The listing builds one solid part. Answer for the finished solid, in the listing's coordinates (mm). Face numbers are marked on the shaded views. A direction names the side the tool comes from. Coordinates: 2 decimals unless noted, no trailing zeros. Write each loop counter-clockwise with the first axis right and the second up, starting at its lowest first coordinate (ties: lowest second). Pieces come first, ordered by that corner, then holes.
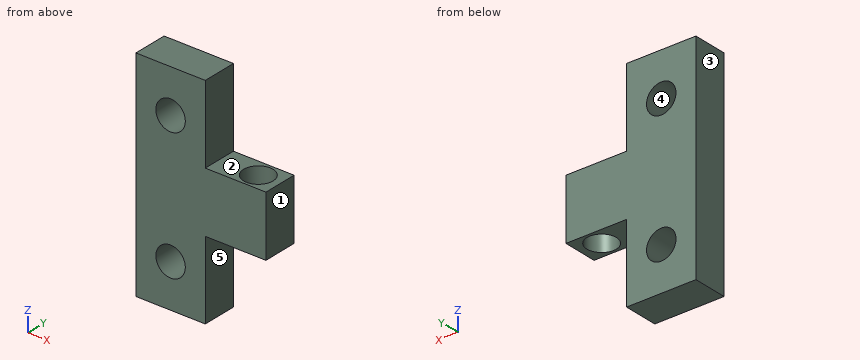
Autodesk Inventor part; units mm, degrees
ref_plane "YZ Plane" through (0, 0, 0) normal (1, 0, 0) x (0, 1, 0)
ref_plane "XZ Plane" through (0, 0, 0) normal (0, 1, 0) x (-1, 0, 0)
ref_plane "XY Plane" through (0, 0, 0) normal (0, 0, 1) x (1, 0, 0)
sketch "Skizze1" plane through (0, 0, 0) normal (0, 1, 0) x (-1, 0, 0)
  line L0 (0, 0) -> (15, 0)
  line L1 (15, 0) -> (15, -25)
  line L2 (15, -25) -> (0, -25)
  line L3 (0, -25) -> (0, 0)
  dimension "d0" = 25
  dimension "d1" = 15
extrude "Extrusion1" add sketch "Skizze1" along normal blind 4
sketch "Skizze3" plane through (0, 0, -25) normal (0, 0, -1) x (-1, 0, 0)
  point P0 (0, 0)
sketch "Skizze6" plane through (0, 4, 0) normal (0, 1, 0) x (1, 0, 0)
  circle A0 centre (-11, 5) radius 1.7
  line L0 (-15, 25) -> (-15, 0)
  line L1 (-15, 0) -> (0, 0)
  circle A1 centre (-11, 20) radius 1.7
  line L2 (0, 25) -> (-15, 25)
  point P0 (0, 30)
  dimension "d11" = 3.4
  dimension "d12" = 4
  dimension "d13" = 5
  dimension "d14" = 3.4
  dimension "d15" = 4
  dimension "d16" = 5
extrude "Extrusion4" cut sketch "Skizze6" against normal blind 30
sketch "Skizze7" plane through (0, 0, 0) normal (0, -1, 0) x (1, 0, 0)
  line L0 (0, -25) -> (-15, -25)
  line L1 (0, -25) -> (-7, -25)
  line L2 (-7, -25) -> (-7, -16)
  line L3 (-7, -16) -> (0, -16)
  line L4 (0, -16) -> (0, -25)
  line L5 (-15, 0) -> (0, 0)
  line L6 (0, 0) -> (-7, 0)
  line L7 (-7, 0) -> (-7, -9)
  line L8 (-7, -9) -> (0, -9)
  line L9 (0, -9) -> (0, 0)
  dimension "d19" = 7
  dimension "d20" = 9
  dimension "d21" = 7
  dimension "d22" = 9
extrude "Extrusion5" cut sketch "Skizze7" against normal blind 30
sketch "Skizze8" plane through (-7, 0, -9) normal (0, 0, 1) x (1, 0, 0)
  circle A0 centre (4.5, 2) radius 1.7
  line L0 (7, 0) -> (0, 0)
  line L1 (7, 4) -> (7, 0)
  dimension "d25" = 3.4
  dimension "d26" = 2
  dimension "d27" = 2.5
extrude "Extrusion6" cut sketch "Skizze8" against normal blind 30
properties part number "kamera ut"
1. A tool of negligible diameter and unlimited length cuts with its end or side. For the marked faces 1 and 2, from which of +Z, -Z, +X, -X, +Y, -Y can it reach the whole face along a straight path? Write none if from no direction.
Results found:
face 1: +Z, -Z, +X, +Y, -Y
face 2: +Z, +X, +Y, -Y
2. Section A-A on y = 2 is taken. Give the vertices of the cut face in (x, z).
Results found:
outline: (-15, -25) - (-7, -25) - (-7, -16) - (-4.2, -16) - (-4.2, -9) - (-7, -9) - (-7, 0) - (-15, 0) - close; (-0.8, -16) - (0, -16) - (0, -9) - (-0.8, -9) - close; hole circle Ø3.4 at (-11, -20); hole circle Ø3.4 at (-11, -5)
3. Section B-B on x = -11 is taken. Give the vertices of the cut face in (y, z).
Results found:
outline: (0, -25) - (4, -25) - (4, -21.7) - (0, -21.7) - close; (0, -18.3) - (4, -18.3) - (4, -6.7) - (0, -6.7) - close; (0, -3.3) - (4, -3.3) - (4, 0) - (0, 0) - close
4. Flat-ended cylindrical pins translate along their axes: P1, Ø1.2, axis at x = -5, y = 1.5, coming from the +Z side; P2, Ø3, axis at x = -11, z = -5, coming from the +Y side; P3, Ø1.2, axis at y = 2.5, z = -4, coming from the +X side. Find the tip coordinate at first contact, or state that the pin passes through.
Results found:
P1: stops at z = -9
P2: passes through
P3: stops at x = -7
5. Find the intervals of material crossed by L1, parallel to Z at x = -11, y = 2.4; L2, parallel to Y at x = -2.5, z = -13.5; L3, parallel to X at y = 1, z = -20, in increasing order.
Results found:
L1: z = -25 to -21.7, -18.3 to -6.7, -3.3 to 0
L2: y = 0 to 0.3, 3.7 to 4
L3: x = -15 to -12.7, -9.3 to -7
6. Section C-C on z = -20 is taken. Give the vertices of the cut face in (x, y).
Results found:
outline: (-15, 0) - (-12.7, 0) - (-12.7, 4) - (-15, 4) - close; (-9.3, 0) - (-7, 0) - (-7, 4) - (-9.3, 4) - close
7. Section D-D on x = -2.5 is taken. Give the vertices of the cut face in (y, z).
Results found:
outline: (0, -16) - (0.3, -16) - (0.3, -9) - (0, -9) - close; (3.7, -16) - (4, -16) - (4, -9) - (3.7, -9) - close
8. For a pull along X with two mould halves and no side action, classify the marked faces 3, 4 and 5 as pulls with the +X half, pulls with the -X half, needs draft (parallel to the pull), parting line crosses it, or undercut.
Results found:
face 3: pulls with the -X half
face 4: undercut
face 5: pulls with the +X half
